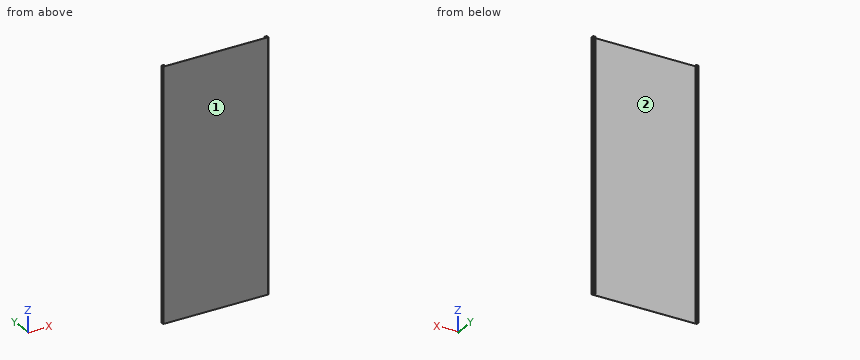
Autodesk Inventor part; units mm, degrees
ref_plane "YZ Plane" through (0, 0, 0) normal (1, 0, 0) x (0, 1, 0)
ref_plane "XZ Plane" through (0, 0, 0) normal (0, 1, 0) x (-1, 0, 0)
ref_plane "XY Plane" through (0, 0, 0) normal (0, 0, 1) x (1, 0, 0)
sketch "Sketch6" plane through (0, 0, 0) normal (0, 1, 0) x (-1, 0, 0)
  line L0 (205.5, -490) -> (-205.5, -490)
  line L1 (-205.5, -490) -> (-205.5, 490)
  line L2 (-205.5, 490) -> (205.5, 490)
  line L3 (205.5, 490) -> (205.5, -490)
  line L4 (205.5, -490) -> (-205.5, 490) construction
  line L5 (-205.5, -490) -> (205.5, 490) construction
  point P0 (0, 0)
  dimension "d52" = 411
  dimension "d53" = 980
extrude "Plate2" add sketch "Sketch6" along normal blind 0.5
sketch "Sketch11" plane through (-205, 0, 490) normal (-1, 0, 0) x (0, -1, 0)
  line L0 (0, -980) -> (0, 0)
  line L1 (0, 0) -> (-10, 0)
  line L2 (-10, 0) -> (-10, -980)
  line L3 (-10, -980) -> (0, -980)
edge flange "Flange2" height 10 angle 90 thickness 0.5 bend radius 0.5 thickness toward (-1, 0, 0) relief tear relief width 0.5 relief depth 0.25 edges at (-205.5, 0.5, 0) wall of the first edge with corners at (-205, 0, -490) (-205, 0, 490) (-205, 10, 490) (-205, 10, -490)
bend "Bend3"
corner "Corner3"
sketch "Sketch12" plane through (-205.5, 9.5, 490) normal (0, 1, 0) x (-1, 0, 0)
  line L0 (0, -980) -> (0, 0)
  line L1 (0, 0) -> (-10, 0)
  line L2 (-10, 0) -> (-10, -980)
  line L3 (-10, -980) -> (0, -980)
edge flange "Flange3" height 10 angle 90 thickness 0.5 bend radius 0.5 thickness toward (0, 1, 0) relief tear relief width 0.5 relief depth 0.25 edges at (-205, 10, 0) wall of the first edge with corners at (-205.5, 9.5, -490) (-205.5, 9.5, 490) (-195.5, 9.5, 490) (-195.5, 9.5, -490)
bend "Bend4"
corner "Corner4"
sketch "Sketch13" plane through (205, 0, -490) normal (1, 0, 0) x (0, 1, 0)
  line L0 (0, 980) -> (0, 0)
  line L1 (0, 0) -> (10, 0)
  line L2 (10, 0) -> (10, 980)
  line L3 (10, 980) -> (0, 980)
edge flange "Flange4" height 10 angle 90 thickness 0.5 bend radius 0.5 thickness toward (1, 0, 0) relief tear relief width 0.5 relief depth 0.25 edges at (205.5, 0.5, 0) wall of the first edge with corners at (205, 0, 490) (205, 0, -490) (205, 10, -490) (205, 10, 490)
bend "Bend5"
corner "Corner5"
sketch "Sketch14" plane through (205.5, 9.5, -490) normal (0, 1, 0) x (-1, 0, 0)
  line L0 (0, 980) -> (0, 0)
  line L1 (0, 0) -> (10, 0)
  line L2 (10, 0) -> (10, 980)
  line L3 (10, 980) -> (0, 980)
edge flange "Flange5" height 10 angle 90 thickness 0.5 bend radius 0.5 thickness toward (0, 1, 0) relief tear relief width 0.5 relief depth 0.25 edges at (205, 10, 0) wall of the first edge with corners at (205.5, 9.5, 490) (205.5, 9.5, -490) (195.5, 9.5, -490) (195.5, 9.5, 490)
bend "Bend6"
corner "Corner6"
equation "\"d52\" = ЖАБРЫ_базовая_ширина - 5 * ЖАБРЫ_шаг_листов"
equation "\"d53\" = ЖАБРЫ_базовая_длина_кор_лист"
equation "\"d54\" = Thickness"
equation "\"d84\" = BendReliefWidth"
equation "\"d85\" = BendReliefDepth"
equation "\"d86\" = MinimumRemnant"
equation "\"d87\" = TransitionRadius"
equation "\"d90\" = BendRadius"
equation "\"d91\" = CornerReliefSize"
equation "\"d92\" = GapSize"
equation "\"d93\" = JacobiRadiusSize"
equation "\"d94\" = BendReliefWidth"
equation "\"d95\" = BendReliefDepth"
equation "\"d96\" = MinimumRemnant"
equation "\"d97\" = TransitionRadius"
equation "\"d100\" = BendRadius"
equation "\"d101\" = CornerReliefSize"
equation "\"d102\" = GapSize"
equation "\"d103\" = JacobiRadiusSize"
equation "\"d104\" = BendReliefWidth"
equation "\"d105\" = BendReliefDepth"
equation "\"d106\" = MinimumRemnant"
equation "\"d107\" = TransitionRadius"
equation "\"d110\" = BendRadius"
equation "\"d111\" = CornerReliefSize"
equation "\"d112\" = GapSize"
equation "\"d113\" = JacobiRadiusSize"
equation "\"d114\" = BendReliefWidth"
equation "\"d115\" = BendReliefDepth"
equation "\"d116\" = MinimumRemnant"
equation "\"d117\" = TransitionRadius"
equation "\"d120\" = BendRadius"
equation "\"d121\" = CornerReliefSize"
equation "\"d122\" = GapSize"
equation "\"d123\" = JacobiRadiusSize"
equation "\"BendRadius\" = Thickness"
equation "\"BendReliefWidth\" = Thickness"
equation "\"BendReliefDepth\" = 0.5 * Thickness"
equation "\"CornerReliefSize\" = 4 * Thickness"
equation "\"MinimumRemnant\" = 2 * Thickness"
equation "\"TransitionRadius\" = BendRadius"
equation "\"JacobiRadiusSize\" = BendRadius"
equation "\"GapSize\" = Thickness"
properties part number "MSC 811 sheet gills" material "Stainless Steel"
Source: CAD feature listing. Evaluate the final solid. Frame: model axes, mm. Face numbers are marked on the shaded views. Round coordinates to 2 decimals unless told otherwise and drop trailing zeros. Loops run counter-clockwise (first coordinate to the right, second up) from the corner with the lowest first, then second, coordinate; pieces in that order, holes last.
Q1. Section C-C, the plane x = -56.5. Return loops of the section in (y, z), plus the area to 3 significant figures.
Q2. Ray query, line 1 (X direction, y = 9.25, z = -26.5); line 2 (X direction, y = 3.5, z = -200.5); line 3 (Y direction, x = 117.5, z = 128). Return the intervals inside material, ascending.
Q3. Mould query, pull axis X, two halves, no side actions, for the marked faces 1 and 2. Classes: pulls with the +X half, pulls with the -X half, needs draft (parallel to the pull), parting line crosses it, or undercut.
Q4. Section B-B, the plane z = 39. Return loops of the section in (x, y).
Q5. Section A-A, the plane y = 3. Return loops of the section in (x, z).
Q6. First-contact query: P1, Ø6, axis at x = -17, z = -142, coming from the +Y side. Flat tip, straight axial feed; report the tip coordinate or a pass-through.
Solutions:
1. outline: (0, -490) - (0.5, -490) - (0.5, 490) - (0, 490) - close
1. area: 490 mm2
2. line 1: x = -205.47 to -204.93, 204.93 to 205.47
2. line 2: x = -205.5 to -205, 205 to 205.5
2. line 3: y = 0 to 0.5
3. face 1: needs draft
3. face 2: undercut
4. outline: (-205.5, 1) arc R1 ccw to (-204.5, 0) - (204.5, 0) arc R1 ccw to (205.5, 1) - (205.5, 9) arc R1 ccw to (204.5, 10) - (195.5, 10) - (195.5, 9.5) - (204.5, 9.5) arc R0.5 cw to (205, 9) - (205, 1) arc R0.5 cw to (204.5, 0.5) - (-204.5, 0.5) arc R0.5 cw to (-205, 1) - (-205, 9) arc R0.5 cw to (-204.5, 9.5) - (-195.5, 9.5) - (-195.5, 10) - (-204.5, 10) arc R1 ccw to (-205.5, 9) - close
5. outline: (-205.5, -490) - (-205, -490) - (-205, 490) - (-205.5, 490) - close; (205, -490) - (205.5, -490) - (205.5, 490) - (205, 490) - close
6. P1: stops at y = 0.5
